Check sheet for the modelled part. Datum: model origin and axes. Units: mm. A direction names the side the tool comes from. Round coordinates to 2 decimals unless told otherwise and drop trailing zeros. Order: outer loops, then holes, each group sorted by start corner. A loop starts at its lowest first (then second) coordinate and runs counter-clockwise, first axis right, second up.
(1) Sectioned sample at A-A, the plane y = 2. Enter the section's corners in (x, z).
(2) Tool access check on faces 1 (the flat face through (0, 0, -3.45)), 2 (the cylindrical face through (3.014, -2.754, 4.285)), 3 (the flat face through (3, 0, -1)). Record the directions out of +Z, -Z, +X, -X, +Y, -Y that give a thin tool (end or side, any length) a straight path to the whole face; none if there is none.
(3) Sectioned sample at C-C, the plane x = 1. Enter the section's corners in (y, z).
(4) Sectioned sample at B-B, the plane z = -4. Enter the section's corners in (x, y).
(5) Thickness scan on probe 1 along X at (y, z) = (-2, 0); probe 2 along Z at (x, y) = (-1.25, 0.5). Record the ranges inside material, lowest first.
(6) Depth check by flat-ended pin: pin 1 (0.7 mm diameter, centred on x = 1.5, z = -2.5, fed in from -Y); pin 2 (2 mm diameter, centred on y = -3, z = 3, fed in from -X); pin 3 (1 mm diameter, centred on y = 1.5, z = 0, fed in from +X). Enter the tip coordinate at first touch or a pass-through.
(7) Sectioned sample at D-D, the plane z = -2. Enter the section's corners in (x, y), and give its area (3 significant figures).
```python
from build123d import *

# Parameters (mm, degrees)
F1_DEPTH  = 6
F2_R      = 0.4
F3_DEPTH  = 2.5
F4_R      = 0.9
F5_DEPTH  = 0.5
F7_W      = 6
F7_H      = 2.2
F8_DEPTH  = 0.75
F9_R      = 0.4
F10_DEPTH = 1.2
F11_SIZE  = 0.1


with BuildPart() as f1:
    # F0 (on Front) → F1 (new body)
    with BuildSketch(Plane.XZ):
        with BuildLine():
            ThreePointArc((3, 1.25), (1.8027756377, 2.7041634566), (0, 3.25))
            ThreePointArc((0, 3.25), (-1.8027756377, 2.7041634566), (-3, 1.25))
            Line((-3, 1.25), (-3, -1.25))
            ThreePointArc((-3, -1.25), (-1.8027756377, -2.7041634566), (0, -3.25))
            ThreePointArc((0, -3.25), (1.8027756377, -2.7041634566), (3, -1.25))
            Line((3, -1.25), (3, 1.25))
        make_face()
    extrude(amount=-F1_DEPTH)

    # F2 (on face) → F3 (join)
    with BuildSketch(Plane.XZ):
        Circle(F2_R)
    extrude(amount=F3_DEPTH)

    # F4 (on face) → F5 (join)
    with BuildSketch(Plane.XZ):
        with BuildLine():
            ThreePointArc((4.7492643315, 3.2614396069), (2.8637824638, 2.8637824638), (3.2614396069, 4.7492643315))
            Line((3.2614396069, 4.7492643315), (-1.1742833736, 3.0304386743))
            ThreePointArc((-1.1742833736, 3.0304386743), (1.2750689268, 2.9894312556), (3, 1.25))
            Line((3, 1.25), (3, -1.25))
            Line((3, -1.25), (4.7492643315, 3.2614396069))
        make_face()
        with BuildLine():
            ThreePointArc((4.7492643315, 3.2614396069), (4.8073656809, 3.4655970706), (4.8269552622, 3.6769552622))
            ThreePointArc((4.8269552622, 3.6769552622), (4.3268233243, 4.6257289453), (3.2614396069, 4.7492643315))
            ThreePointArc((3.2614396069, 4.7492643315), (2.8637824638, 2.8637824638), (4.7492643315, 3.2614396069))
        make_face()
        with Locations((3.6769552622, 3.6769552622)):
            Circle(F4_R, mode=Mode.SUBTRACT)
    extrude(amount=-F5_DEPTH)


with BuildPart() as f1_1:
    # F6: moved
    add(f1.part.moved(Location((0, -3, 0))))

    # F7 (on Front) → F8 (join, symmetric)
    with BuildSketch(Plane.XZ):
        with Locations((0, -2.35)):
            Rectangle(F7_W, F7_H)
    extrude(amount=F8_DEPTH, both=True)

    # F9 (on face) → F10 (join)
    with BuildSketch(Plane(origin=(0, 0, -3.45), x_dir=(1, 0, 0), z_dir=(0, 0, -1))):
        with Locations((-2.5, 0)):
            Circle(F9_R)
        with Locations((-1, 0)):
            Circle(F9_R)
        with Locations((1, 0)):
            Circle(F9_R)
        with Locations((2.5, 0)):
            Circle(F9_R)
    extrude(amount=F10_DEPTH)

    # F11
    f11_edges = [f1_1.edges().sort_by_distance(p)[0] for p in [
        (-2.9, 0, -4.65),
        (-1.4, 0, -4.65),
        (0.6, 0, -4.65),
        (2.1, 0, -4.65),
    ]]
    chamfer(f11_edges, length=F11_SIZE)


solid = f1_1.part
```
Derived:
1. outline: (-3, -1.25) arc R3.25 ccw to (3, -1.25) - (3, 1.25) arc R3.25 ccw to (-3, 1.25) - close
2. face 1: -Z
2. face 2: +Y, -Y
2. face 3: +Z, -Z, +X, +Y
3. outline: (-3, -3.09) - (-0.75, -3.09) - (-0.75, -3.45) - (-0.4, -3.45) - (-0.4, -4.55) - (-0.3, -4.65) - (0.3, -4.65) - (0.4, -4.55) - (0.4, -3.45) - (0.75, -3.45) - (0.75, -3.09) - (3, -3.09) - (3, 3.09) - (-2.5, 3.09) - (-2.5, 3.87) - (-3, 3.87) - close
4. outline: circle Ø0.8 at (-2.5, 0); circle Ø0.8 at (-1, 0); circle Ø0.8 at (1, 0); circle Ø0.8 at (2.5, 0)
5. probe 1: x = -3 to 3
5. probe 2: z = -3.45 to 3
6. pin 1: stops at y = -3
6. pin 2: stops at x = -2.56
6. pin 3: stops at x = 3
7. outline: (-3, -0.75) - (-2.56, -0.75) - (-2.56, -3) - (2.56, -3) - (2.56, -0.75) - (3, -0.75) - (3, 0.75) - (2.56, 0.75) - (2.56, 3) - (-2.56, 3) - (-2.56, 0.75) - (-3, 0.75) - close
7. area: 32.1 mm2
